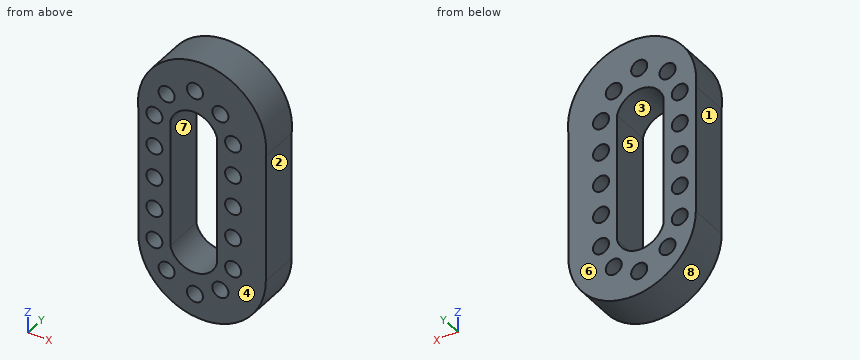
from build123d import *

# Parameters (mm, degrees)
F0_R     = 5
F1_DEPTH = 25


with BuildPart() as f1:
    # F0 (on Front) → F1 (new body)
    with BuildSketch(Plane.XZ):
        with BuildLine():
            ThreePointArc((44.202886, 38.641287), (4.450733, 83.087214), (-35.301421, 38.641287))
            Line((-35.301421, 38.641287), (-35.301421, -41.358713))
            ThreePointArc((-35.301421, -41.358713), (4.450733, -81.110867), (44.202886, -41.358713))
            Line((44.202886, -41.358713), (44.202886, 38.641287))
        make_face()
        with Locations((-17.662896, -57.657674)):
            Circle(F0_R, mode=Mode.SUBTRACT)
        with Locations((-25.301421, -41.358713)):
            Circle(F0_R, mode=Mode.SUBTRACT)
        with Locations((0, -66.3588)):
            Circle(F0_R, mode=Mode.SUBTRACT)
        with Locations((-25.301421, -21.358713)):
            Circle(F0_R, mode=Mode.SUBTRACT)
        with Locations((-25.301421, -1.358713)):
            Circle(F0_R, mode=Mode.SUBTRACT)
        with BuildLine():
            ThreePointArc((-15.301421, 38.641287), (-0.742925, 50.028783), (13.815571, 38.641287))
            Line((13.815571, 38.641287), (13.815571, -41.358713))
            ThreePointArc((13.815571, -41.358713), (-0.742925, -52.746209), (-15.301421, -41.358713))
            Line((-15.301421, -41.358713), (-15.301421, 38.641287))
        make_face(mode=Mode.SUBTRACT)
        with Locations((15.870508, -57.657674)):
            Circle(F0_R, mode=Mode.SUBTRACT)
        with Locations((23.815571, -41.358713)):
            Circle(F0_R, mode=Mode.SUBTRACT)
        with Locations((23.815571, -21.358713)):
            Circle(F0_R, mode=Mode.SUBTRACT)
        with Locations((23.815571, -1.358713)):
            Circle(F0_R, mode=Mode.SUBTRACT)
        with Locations((-25.301421, 18.641287)):
            Circle(F0_R, mode=Mode.SUBTRACT)
        with Locations((-25.301421, 38.641287)):
            Circle(F0_R, mode=Mode.SUBTRACT)
        with Locations((-17.662896, 54.878572)):
            Circle(F0_R, mode=Mode.SUBTRACT)
        with Locations((0, 63.641374)):
            Circle(F0_R, mode=Mode.SUBTRACT)
        with Locations((23.815571, 18.641287)):
            Circle(F0_R, mode=Mode.SUBTRACT)
        with Locations((23.815571, 38.641287)):
            Circle(F0_R, mode=Mode.SUBTRACT)
        with Locations((15.870508, 54.878572)):
            Circle(F0_R, mode=Mode.SUBTRACT)
    extrude(amount=F1_DEPTH)


solid = f1.part
The model under review builds one solid part; all positions refer to its coordinate system, in mm. Face numbers are marked on the shaded views. A direction names the side the tool comes from. Coordinates: 2 decimals unless noted, no trailing zeros. Write each loop counter-clockwise with the first axis right and the second up, starting at its lowest first coordinate (ties: lowest second). Pieces come first, ordered by that corner, then holes. Notation, with made-up numbers: (5.5, 24.25) - (9.5, 24.25) arc R10 ccw to (9.5, 41.25) - close; hole circle Ø9 at (5, -16.75). An arc over 180 degrees is marked (long way). Answer as a JSON object with one key per item and string values. Group by question number.
1. Clearance check with flat-ended pins moving along their axes: pin 1 Ø8 at (x, z) = (-25.3, 18.64) entering from +Y; pin 2 Ø3 at (y, z) = (-15, -10) entering from +X; pin 3 Ø12.5 at (y, z) = (-16.5, -15.5) entering from -X; pin 4 Ø1 at (x, y) = (2.5, -15) entering from -Z. State where each tip first meets the part, or that it passes through.
2. Add section B-B (x = 0). Give the boundary of the cut face in (y, z), plus the area to 3 significant figures.
3. Add section D-D (y = -9.5). Give the number of separate pieces and of enclosed holes in the cut face, plus the area to 3 significant figures.
4. Add section C-C (z = 1). Give the boundary of the cut face in (x, y), plus the area to 3 significant figures.
5. Mouldability with a two-part tool opening along Z and no side actions: class the marked faces 5, 6, 7 and 8 as pulls with the +Z half, pulls with the -Z half, needs draft (parallel to the pull), parting line crosses it, or undercut.
6. Add section A-A (z = -30.5). Give the boundary of the cut face in (x, y), plus the area to 3 significant figures.
7. Machinability: for the marked faces 1, 2, 3 and 4, which of the approach directions +Z, -Z, +X, -X, +Y, -Y give a long, thin tool a straight path to every point of the face, cutting with its end or side? Answer none if there is none.
8. To check wall thickness, follow probe 1 along X at (y, z) = (-10.5, 8.5); probe 2 along Z at (x, y) = (15.5, -15); probe 3 along Z at (x, y) = (-17.5, -3). State the ranges of each line that lie inside material, in increasing order.
Findings:
{
 "1": {"pin 1": "through", "pin 2": "x = 44.2", "pin 3": "x = -35.3", "pin 4": "z = -81.08"},
 "2": {"outline": "(-25, -80.86) - (0, -80.86) - (0, -71.36) - (-25, -71.36) - close; (-25, -61.36) - (0, -61.36) - (0, -52.73) - (-25, -52.73) - close; (-25, 50.01) - (0, 50.01) - (0, 58.64) - (-25, 58.64) - close; (-25, 68.64) - (0, 68.64) - (0, 82.84) - (-25, 82.84) - close", "area": "1,020 mm²"},
 "3": {"separate pieces": "1", "enclosed holes": "17", "area": "7,630 mm²"},
 "4": {"outline": "(-35.3, -25) - (-29.71, -25) - (-29.71, 0) - (-35.3, 0) - close; (-20.89, -25) - (-15.3, -25) - (-15.3, 0) - (-20.89, 0) - close; (13.82, -25) - (19.41, -25) - (19.41, 0) - (13.82, 0) - close; (28.22, -25) - (44.2, -25) - (44.2, 0) - (28.22, 0) - close", "area": "819 mm²"},
 "5": {"face 5": "undercut", "face 6": "needs draft", "face 7": "undercut", "face 8": "pulls with the -Z half"},
 "6": {"outline": "(-35.3, -25) - (-15.3, -25) - (-15.3, 0) - (-35.3, 0) - close; (13.82, -25) - (44.2, -25) - (44.2, 0) - (13.82, 0) - close", "area": "1,260 mm²"},
 "7": {"face 1": "-Z, -X, +Y, -Y", "face 2": "-Z, +X, +Y, -Y", "face 3": "+Y, -Y", "face 4": "+Z, -Z, +X, -X, -Y"},
 "8": {"probe 1": "-35.3 to -15.3, 13.82 to 44.2", "probe 2": "-79.54 to -62.64, -52.67 to 49.89, 59.86 to 81.53", "probe 3": "-74.5 to -62.66, -52.66 to 49.88, 59.88 to 76.53"}
}
